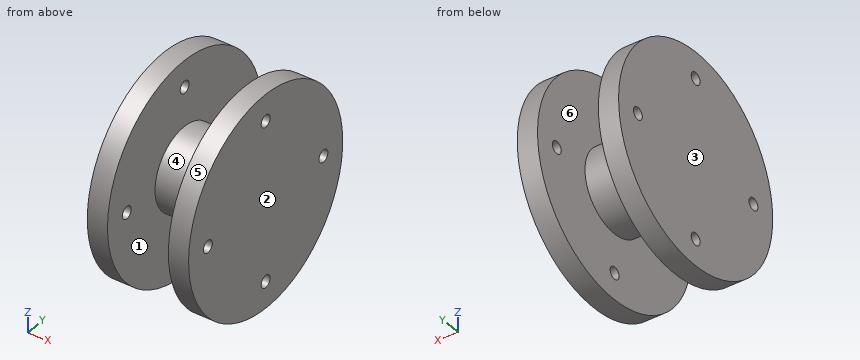
```python
from build123d import *

# Parameters (mm, degrees)
SKETCH_2_R               = 1.5
CUT_EXTRUDE_1_DEPTH      = 45.463468151
PATTERN_CIRCULAR_1_COUNT = 4


with BuildPart() as part:
    # Sketch 1 → Revolve 1 (revolve)
    with BuildSketch(Plane.XY, mode=Mode.PRIVATE) as revolve_1_sk:
        Polygon((0, 0), (0, 26), (5, 26), (5, 10), (20, 10), (20, 26), (25, 26), (25, 0), align=None)
    revolve(revolve_1_sk.sketch.rotate(Axis((0, 0, 0), (1, 0, 0)), 90), axis=Axis((0, 0, 0), (1, 0, 0)))

    # Sketch 2 → Cut-Extrude 1 (cut, through all)
    with BuildSketch(Plane.ZY):
        with Locations((0, 19.5)):
            Circle(SKETCH_2_R)
    cut_extrude_1 = extrude(amount=-CUT_EXTRUDE_1_DEPTH, mode=Mode.SUBTRACT)

    # Pattern Circular 1: Cut-Extrude 1 ×4 about axis
    pattern_circular_1_axis = Axis((0, 0, 0), (1, 0, 0))
    for i in range(1, PATTERN_CIRCULAR_1_COUNT):
        add(cut_extrude_1.rotate(pattern_circular_1_axis, i * 360 / PATTERN_CIRCULAR_1_COUNT), mode=Mode.SUBTRACT)


solid = part.part
```
CAD build for the part. Positions are in the model's coordinates, mm. Face numbers are marked on the shaded views. A direction names the side the tool comes from. Round coordinates to 2 decimals unless told otherwise and drop trailing zeros. Write each loop counter-clockwise with the first axis right and the second up, starting at its lowest first coordinate (ties: lowest second). Pieces come first, ordered by that corner, then holes. Notation, with made-up numbers: (88, -1.5) - (95, -1.5) arc R30 cw to (95, 29.5) - close; hole circle Ø11 at (72.5, -4.75). An arc over 180 degrees is marked (long way). Write item = value, one per line. Start each with the question number.
Q1. Band-saw the part on D-D (x = 2.5). Give the cut face in (y, z).
Q2. Drop flat-ended pins along their axis: pin 1 (5 mm diameter, centred on x = 16.5, z = 11.5, fed in from -Y); pin 2 (3 mm diameter, centred on x = 19, y = 16, fed in from +Z); pin 3 (8 mm diameter, centred on x = 4.5, y = -9.5, fed in from +Z); pin 4 (5 mm diameter, centred on y = 0, z = 19.5, fed in from +X). Give the stop position or say it passes through.
Q3. Band-saw the part on A-A (z = 0). Give the cut face in (x, y), then the cut area to 3 significant figures.
Q4. Mould opens along X. For the marked faces 3, 4, 5 and 6 say: pulls with the +X half, pulls with the -X half, needs draft (parallel to the pull), parting line crosses it, or undercut.
Q5. Which spindle directions (+Z, -Z, +X, -X, +Y, -Y) get a long thin tool onto all of the face, cutting with end or side? Do the marked faces 1 and 2. Say none if no direction does.
Q6. Band-saw the part on C-C (z = -19.5). Give the cut face in (x, y).
Q7. Probe L1, parallel to Y at x = 21.5, z = 0; L2, parallel to X at y = -3, z = 21; L3, parallel to Y at x = 19.25, z = 0. List the from-to ranges inside material, lowest first. Write a range as from..to.
Answers below:
q1.outline = circle Ø52 at (0, 0); hole circle Ø3 at (-19.5, 0); hole circle Ø3 at (0, -19.5); hole circle Ø3 at (0, 19.5); hole circle Ø3 at (19.5, 0)
q2.pin_1 = -4.36
q2.pin_2 = 21.32
q2.pin_3 = 25.41
q2.pin_4 = 25
q3.outline = (0, -26) - (5, -26) - (5, -21) - (0, -21) - close; (0, -18) - (5, -18) - (5, -10) - (20, -10) - (20, -18) - (25, -18) - (25, 18) - (20, 18) - (20, 10) - (5, 10) - (5, 18) - (0, 18) - close; (0, 21) - (5, 21) - (5, 26) - (0, 26) - close; (20, -26) - (25, -26) - (25, -21) - (20, -21) - close; (20, 21) - (25, 21) - (25, 26) - (20, 26) - close
q3.area = 760 mm2
q4.face_3 = pulls with the -X half
q4.face_4 = undercut
q4.face_5 = needs draft
q4.face_6 = undercut
q5.face_1 = none
q5.face_2 = +Z, -Z, +X, +Y, -Y
q6.outline = (0, -17.2) - (5, -17.2) - (5, -1.5) - (0, -1.5) - close; (0, 1.5) - (5, 1.5) - (5, 17.2) - (0, 17.2) - close; (20, -17.2) - (25, -17.2) - (25, -1.5) - (20, -1.5) - close; (20, 1.5) - (25, 1.5) - (25, 17.2) - (20, 17.2) - close
q7.L1 = -26..-21, -18..18, 21..26
q7.L2 = 0..5, 20..25
q7.L3 = -10..10
